```python
from build123d import *

# Parameters (mm, degrees)
SKETCH_1_W                         = 120
SKETCH_1_H                         = 120
EXTRUDE_1_DEPTH                    = 5
SKETCH_2_W                         = 60
SKETCH_2_H                         = 60
SKETCH_2_W_2                       = 54
SKETCH_2_H_2                       = 54
EXTRUDE_2_DEPTH                    = 2000
FILLET_1_R                         = 5
SKETCH_3_R                         = 5
CUT_EXTRUDE_1_DEPTH                = 2000
EXTRUDE_5_DEPTH                    = 7.5
PATTERN_LINEAR_1_COUNT             = 2
PATTERN_LINEAR_1_PITCH             = 1500
SKETCH_7_R                         = 12.5
EXTRUDE_6_DEPTH                    = 30
SKETCH_8_R                         = 4
EXTRUDE_7_DEPTH                    = 35
PATTERN_LINEAR_2_COUNT             = 2
PATTERN_LINEAR_2_PITCH             = 1500
PATTERN_CIRCULAR_2_COUNT           = 2
PATTERN_CIRCULAR_2_ANGLE           = 90
PATTERN_CIRCULAR_2_COPY_1_DEPTH    = 7.5
PATTERN_CIRCULAR_2_COPY_2_SKETCH_R = 12.5
PATTERN_CIRCULAR_2_COPY_2_DEPTH    = 30
PATTERN_CIRCULAR_2_COPY_3_SKETCH_R = 4
PATTERN_CIRCULAR_2_COPY_3_DEPTH    = 35


with BuildPart() as part:
    # Sketch 1 → Extrude 1 (new body)
    with BuildSketch(Plane(origin=(0, 0, 0), x_dir=(1, 0, 0), z_dir=(0, 1, 0))):
        Rectangle(SKETCH_1_W, SKETCH_1_H)
    extrude(amount=EXTRUDE_1_DEPTH)

    # Sketch 2 → Extrude 2 (add)
    with BuildSketch(Plane(origin=(0, 5, 0), x_dir=(1, 0, 0), z_dir=(0, 1, 0))):
        Rectangle(SKETCH_2_W, SKETCH_2_H)
        Rectangle(SKETCH_2_W_2, SKETCH_2_H_2, mode=Mode.SUBTRACT)
    extrude(amount=EXTRUDE_2_DEPTH)

    # Fillet 1
    fillet_1_edges = [part.edges().sort_by_distance(p)[0] for p in [
        (30, 1005, -30),
        (-30, 1005, -30),
        (-30, 1005, 30),
        (30, 1005, 30),
    ]]
    fillet(fillet_1_edges, radius=FILLET_1_R)

    # Sketch 3 → Cut-Extrude 1 (cut)
    with BuildSketch(Plane(origin=(0, 5, 0), x_dir=(1, 0, 0), z_dir=(0, 1, 0))):
        with Locations(Location((-45, 45, 0), (0, 0, 270))):
            Circle(SKETCH_3_R)
        with Locations(Location((45, 45, 0), (0, 0, 270))):
            Circle(SKETCH_3_R)
        with Locations(Location((-45, -45, 0), (0, 0, 270))):
            Circle(SKETCH_3_R)
        with Locations(Location((45, -45, 0), (0, 0, 270))):
            Circle(SKETCH_3_R)
    extrude(amount=-CUT_EXTRUDE_1_DEPTH, mode=Mode.SUBTRACT)

    # Sketch 6 → Extrude 5 (add, symmetric)
    with BuildSketch(Plane(origin=(0, 0, 0), x_dir=(0, 0, -1), z_dir=(1, 0, 0))):
        Polygon((30, 1785), (30, 1725), (40, 1725), (40, 1755), (33, 1755), (33, 1785), align=None)
    extrude_5 = extrude(amount=EXTRUDE_5_DEPTH, both=True)

    # Pattern Linear 1: Extrude 5 ×2
    with Locations(*[(0, -i * PATTERN_LINEAR_1_PITCH, 0) for i in range(1, PATTERN_LINEAR_1_COUNT)]):
        add(extrude_5)

    # Sketch 7 → Extrude 6 (add)
    with BuildSketch(Plane(origin=(0, 1755, 0), x_dir=(1, 0, 0), z_dir=(0, 1, 0))):
        with Locations((0, 52)):
            Circle(SKETCH_7_R)
    extrude_6 = extrude(amount=-EXTRUDE_6_DEPTH)

    # Sketch 8 → Extrude 7 (add)
    with BuildSketch(Plane(origin=(0, 1755, 0), x_dir=(1, 0, 0), z_dir=(0, 1, 0))):
        with Locations(Location((0, 50, 0), (0, 0, 90))):
            Circle(SKETCH_8_R)
    extrude_7 = extrude(amount=EXTRUDE_7_DEPTH)

    # Pattern Linear 2: Extrude 6, Extrude 7 ×2
    with Locations(*[(0, -i * PATTERN_LINEAR_2_PITCH, 0) for i in range(1, PATTERN_LINEAR_2_COUNT)]):
        add(extrude_6)
        add(extrude_7)

    # Pattern Circular 2: Extrude 5, Extrude 6, Extrude 7 ×2 about axis
    pattern_circular_2_axis = Axis((0, 0, 0), (0, -1, 0))
    add([extrude_5.rotate(pattern_circular_2_axis, i * PATTERN_CIRCULAR_2_ANGLE / (PATTERN_CIRCULAR_2_COUNT - 1)) for i in range(1, PATTERN_CIRCULAR_2_COUNT)])
    add([extrude_6.rotate(pattern_circular_2_axis, i * PATTERN_CIRCULAR_2_ANGLE / (PATTERN_CIRCULAR_2_COUNT - 1)) for i in range(1, PATTERN_CIRCULAR_2_COUNT)])
    add([extrude_7.rotate(pattern_circular_2_axis, i * PATTERN_CIRCULAR_2_ANGLE / (PATTERN_CIRCULAR_2_COUNT - 1)) for i in range(1, PATTERN_CIRCULAR_2_COUNT)])

    # Pattern Circular 2 copy 1 sketch → Pattern Circular 2 copy 1 (add, symmetric)
    with BuildSketch(Plane(origin=(0, -1500, 0), x_dir=(1, 0, 0), z_dir=(0, 0, 1))):
        Polygon((30, 1785), (30, 1725), (40, 1725), (40, 1755), (33, 1755), (33, 1785), align=None)
    extrude(amount=PATTERN_CIRCULAR_2_COPY_1_DEPTH, both=True)

    # Pattern Circular 2 copy 2 sketch → Pattern Circular 2 copy 2 (add)
    with BuildSketch(Plane.ZX.offset(255)):
        with Locations((0, 52)):
            Circle(PATTERN_CIRCULAR_2_COPY_2_SKETCH_R)
    extrude(amount=-PATTERN_CIRCULAR_2_COPY_2_DEPTH)

    # Pattern Circular 2 copy 3 sketch → Pattern Circular 2 copy 3 (add)
    with BuildSketch(Plane.ZX.offset(255)):
        with Locations(Location((0, 50, 0), (0, 0, 90))):
            Circle(PATTERN_CIRCULAR_2_COPY_3_SKETCH_R)
    extrude(amount=PATTERN_CIRCULAR_2_COPY_3_DEPTH)


solid = part.part
```
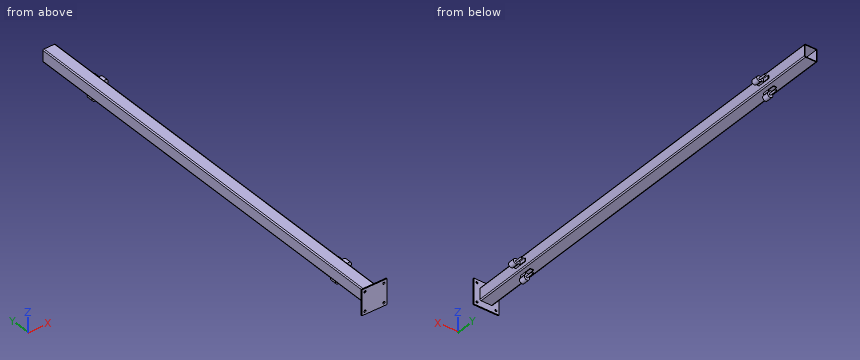
Input: part model. Units: mm. Frame: model coordinates. Coordinates: 2 decimals unless noted, no trailing zeros. Loops run counter-clockwise (first coordinate to the right, second up) from the corner with the lowest first, then second, coordinate; pieces in that order, holes last. Notation, with made-up numbers: M 51,-21 L 87,-21 A17 cw 87,-4 Z; hole C -10.75,49.25 d1. An arc over 180 degrees is marked long. One line per item, written item: value.
(1) Section A-A (y = 561). Output: boundary loops of the cut face in (x, z), and give its area (3 significant figures).
Filled in:
outline: M -30,-25 A5 ccw -25,-30 L 25,-30 A5 ccw 30,-25 L 30,25 A5 ccw 25,30 L -25,30 A5 ccw -30,25 Z; hole M -27,-27 L 27,-27 L 27,27 L -27,27 Z
area: 663 mm^2
(2) Line query: line 1 along X through (y, z) = (2, -45); line 2 along Y through (x, z) = (32, -0.5); line 3 along Y through (x, z) = (45.5, -8). Output: solid intervals per line, ascending. Write a range as from..to.
Filled in:
line 1: -60..-50, -40..40, 50..60
line 2: 0..5, 225..285, 1725..1785
line 3: 0..5, 225..255, 1725..1755
(3) Pin query (flat end, axial travel): pin 1 (8 mm diameter, centred on x = -42.5, z = 7, fed in from -Y); pin 2 (16 mm diameter, centred on x = -5.5, y = 1364.5, fed in from +Z); pin 3 (5 mm diameter, centred on y = 245, z = -34.5, fed in from -X); pin 4 (7.5 mm diameter, centred on x = 1, y = 1768.5, fed in from -Z). Return the tip coordinate at first contact, or that it passes through.
Filled in:
pin 1: y = 0
pin 2: z = 30
pin 3: x = -7.5
pin 4: z = -54
